from build123d import *

# Parameters (mm, degrees)
SKETCH_W               = 190
SKETCH_H               = 100
PAD_DEPTH              = 10
SKETCH001_R            = 2.5
HOLE_DEPTH             = 10.001
SKETCH002_R            = 2.5
HOLE001_DEPTH          = 10.001
LINEARPATTERN_COUNT    = 2
LINEARPATTERN_PITCH    = 15
LINEARPATTERN001_COUNT = 2
LINEARPATTERN001_PITCH = 70
LINEARPATTERN002_COUNT = 2
LINEARPATTERN002_PITCH = 85
LINEARPATTERN003_COUNT = 2
LINEARPATTERN003_PITCH = 130


with BuildPart() as part:
    # Sketch → Pad (new body)
    with BuildSketch(Plane.XY):
        with Locations((95, 50)):
            Rectangle(SKETCH_W, SKETCH_H)
    extrude(amount=PAD_DEPTH)

    # Sketch001 (on Face6 of Pad) → Hole (cut, through all)
    with BuildSketch(Plane.XY.offset(10)):
        with Locations((7.5, 10)):
            Circle(SKETCH001_R)
    extrude(amount=-HOLE_DEPTH, mode=Mode.SUBTRACT)

    # Sketch002 (on Face5 of Hole) → Hole001 (cut, through all)
    with BuildSketch(Plane.XY.offset(10)):
        with Locations((52.5, 10)):
            Circle(SKETCH002_R)
    hole001 = extrude(amount=-HOLE001_DEPTH, mode=Mode.SUBTRACT)

    # LinearPattern: Hole001 ×2
    with Locations(*[(i * LINEARPATTERN_PITCH, 0, 0) for i in range(1, LINEARPATTERN_COUNT)]):
        add(hole001, mode=Mode.SUBTRACT)

    # LinearPattern001: Hole001 ×2
    with Locations(*[(i * LINEARPATTERN001_PITCH, 0, 0) for i in range(1, LINEARPATTERN001_COUNT)]):
        add(hole001, mode=Mode.SUBTRACT)

    # LinearPattern002: Hole001 ×2
    with Locations(*[(i * LINEARPATTERN002_PITCH, 0, 0) for i in range(1, LINEARPATTERN002_COUNT)]):
        add(hole001, mode=Mode.SUBTRACT)

    # LinearPattern003: Hole001 ×2
    with Locations(*[(i * LINEARPATTERN003_PITCH, 0, 0) for i in range(1, LINEARPATTERN003_COUNT)]):
        add(hole001, mode=Mode.SUBTRACT)


solid = part.part
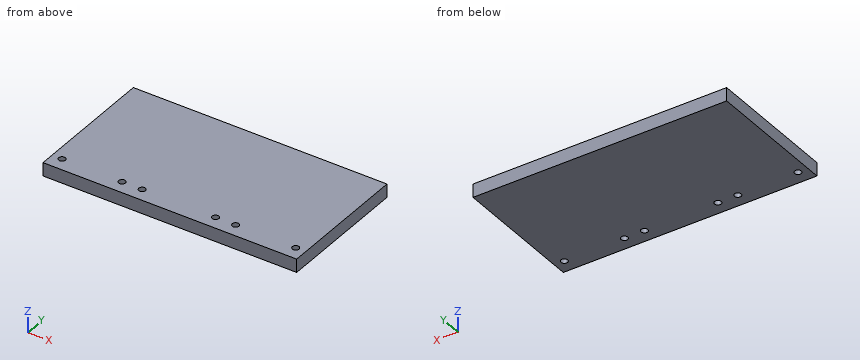
Work out the finished part from the listing and answer in its coordinate system (mm). Coordinates: 2 decimals unless noted, no trailing zeros. Write each loop counter-clockwise with the first axis right and the second up, starting at its lowest first coordinate (ties: lowest second). Pieces come first, ordered by that corner, then holes.
1. The part is cut by section A-A, the plane x = 7.5. Write down the section's boundary in (y, z), and give its area (3 significant figures).
Results list:
outline: (0, 0) - (7.5, 0) - (7.5, 10) - (0, 10) - close; (12.5, 0) - (100, 0) - (100, 10) - (12.5, 10) - close
area: 950 mm2
2. The part is cut by section B-B, the plane y = 10. Write down the section's boundary in (x, z), and give its area (3 significant figures).
Results list:
outline: (0, 0) - (5, 0) - (5, 10) - (0, 10) - close; (10, 0) - (50, 0) - (50, 10) - (10, 10) - close; (55, 0) - (65, 0) - (65, 10) - (55, 10) - close; (70, 0) - (120, 0) - (120, 10) - (70, 10) - close; (125, 0) - (135, 0) - (135, 10) - (125, 10) - close; (140, 0) - (180, 0) - (180, 10) - (140, 10) - close; (185, 0) - (190, 0) - (190, 10) - (185, 10) - close
area: 1,600 mm2
3. Consider line 1 along Y through (x, z) = (7.5, 4.25); line 2 along Y through (x, z) = (8.5, 5.75). Determine where each line is inside the solid, lowest interval first.
Results list:
line 1: y = 0 to 7.5, 12.5 to 100
line 2: y = 0 to 7.71, 12.29 to 100
4. Flat-ended cylindrical pins translate along their axes: pin 1 (4.5 mm diameter, centred on x = 67.5, y = 10, fed in from +Z); pin 2 (6 mm diameter, centred on y = 44.5, z = 2.5, fed in from -X). Find the tip coordinate at first contact, or state that the pin passes through.
Results list:
pin 1: passes through
pin 2: stops at x = 0
